Autodesk Inventor part; units mm, degrees
ref_plane "YZ Plane" through (0, 0, 0) normal (1, 0, 0) x (0, 1, 0)
ref_plane "XZ Plane" through (0, 0, 0) normal (0, 1, 0) x (-1, 0, 0)
ref_plane "XY Plane" through (0, 0, 0) normal (0, 0, 1) x (1, 0, 0)
sketch "草圖1" plane through (0, 0, 0) normal (0, 1, 0) x (-1, 0, 0)
  line L0 (-33.5, 27) -> (33.5, 27)
  line L1 (33.5, 27) -> (33.5, -27)
  line L2 (33.5, -27) -> (-33.5, -27)
  line L3 (-33.5, -27) -> (-33.5, 27)
  line L4 (-33.5, 27) -> (33.5, -27) construction
  line L5 (33.5, 27) -> (-33.5, -27) construction
  line L6 (43.5, -4.5) -> (33.5, -4.5)
  line L7 (33.5, -4.5) -> (33.5, 4.5)
  line L8 (33.5, 4.5) -> (43.5, 4.5)
  line L9 (43.5, 4.5) -> (43.5, -4.5)
  line L10 (-33.5, -4.5) -> (-43.5, -4.5)
  line L11 (-43.5, -4.5) -> (-43.5, 4.5)
  line L12 (-43.5, 4.5) -> (-33.5, 4.5)
  line L13 (-33.5, 4.5) -> (-33.5, -4.5)
  point P0 (0, 0)
  point P1 (33.5, 0)
  point P2 (-33.5, 0)
  point P3 (-33.5, 4.5)
  point P4 (-33.5, -4.5)
  dimension "d0" = 67
  dimension "d1" = 54
  dimension "d2" = 9
  dimension "d3" = 10
extrude "擠出1" add sketch "草圖1" along normal blind 450
sketch "草圖2" plane through (-33.5, 0, 27) normal (0, 0, 1) x (1, 0, 0)
  line L0 (0, 0) -> (0, 450)
  line L1 (0, 450) -> (67, 450)
  line L2 (67, 450) -> (67, 0)
  line L3 (67, 0) -> (0, 0)
  circle A0 centre (33.5, 225) radius 30
  line L4 (3.5, 225) -> (63.5, 225)
  line L5 (63.5, 225) -> (63.5, -27.0162)
  line L6 (63.5, -27.0162) -> (3.5, -27.0162)
  line L7 (3.5, -27.0162) -> (3.5, 225)
  point P0 (33.5, 0)
  point P1 (33.5, 0)
  point P2 (63.5, 225)
  point P3 (3.5, 225)
  dimension "d6" = 225
  dimension "d7" = 60
extrude "擠出2" cut sketch "草圖2" against normal through all contours L7 A0 L5 L3 | L3 L5 L6 L7 | L4 A0 | A0 L4
sketch "草圖3" plane through (-33.5, 450, 27) normal (0, 0, 1) x (1, 0, 0)
  line L0 (-76.6135, -320) -> (143.6135, -320)
  line L1 (143.6135, -320) -> (143.6135, -450)
  line L2 (143.6135, -450) -> (-76.6135, -450)
  line L3 (-76.6135, -450) -> (-76.6135, -320)
  point P0 (33.5, -450)
  point P1 (33.5, -450)
  dimension "d10" = 130
extrude "擠出3" cut sketch "草圖3" against normal through all
sketch "草圖4" plane through (33.5, 450, -27) normal (0, 0, -1) x (-1, 0, 0)
  arc A0 (63.5, -225) -> (3.5, -225) centre (33.5, -225) ccw construction
  circle A1 centre (33.5, -193) radius 30
  line L0 (63.5, -320) -> (3.5, -320)
  line L1 (3.5, -320) -> (3.5, -193)
  line L2 (3.5, -193) -> (63.5, -193)
  line L3 (63.5, -193) -> (63.5, -320)
  point P0 (33.5, -450)
  point P1 (63.5, -320)
  dimension "d13" = 32
  dimension "d14" = 60
sketch "草圖5" plane through (-33.5, 450, 27) normal (0, 0, 1) x (1, 0, 0)
  circle A0 centre (33.5, -191) radius 30
  arc A1 (63.5, -225) -> (3.5, -225) centre (33.5, -225) ccw construction
  line L0 (63.5, -320) -> (3.5, -320)
  line L1 (3.5, -320) -> (3.5, -191)
  line L2 (3.5, -191) -> (63.5, -191)
  line L3 (63.5, -191) -> (63.5, -320)
  point P0 (33.5, -450)
  point P1 (63.5, -320)
  dimension "d15" = 34
  dimension "d16" = 60
loft "斷面混成1" cut profiles "草圖4", "草圖5"
properties part number "Slider-9"
CAD build for the part. Positions are in the model's coordinates, mm. A direction names the side the tool comes from. Round coordinates to 2 decimals unless told otherwise and drop trailing zeros. Order: outer loops, then holes, each group sorted by start corner. A loop starts at its lowest first (then second) coordinate and runs counter-clockwise, first axis right, second up.
Q1. Drop flat-ended pins along their axis: pin 1 (10 mm diameter, centred on y = 392, z = -13, fed in from +X); pin 2 (11 mm diameter, centred on y = 350, z = 13.5, fed in from -X); pin 3 (3 mm diameter, centred on x = -37.5, y = 254.5, fed in from +Z). Give the stop position or say it passes through.
Q2. Slice it at C-C (x = -36.5). Write the cut outline in (y, z), and give its area (3 significant figures).
Q3. Which spindle directions (+Z, -Z, +X, -X, +Y, -Y) get a long thin tool onto all of the face, cutting with end or side? Do faces 4 (the flat face through (30, 195, 0)), 5 (the flat face through (-38, 288, 4.5)), 6 (the flat face through (-39, 288, -4.5)). Say none if no direction does.
Q4. Two-plate mould, pull along X, no slides. Class faces 1 (the flat face through (33.5, 288, -16)), 2 (the flat face through (0, 359, -27)), 3 (the flat face through (-30, 194, 0)): pulls with the +X half, pulls with the -X half, needs draft (parallel to the pull), parting line crosses it, or undercut.
Q5. Slice it at A-A (y = 215). Write the cut outline in (x, z).
Q6. Wall check: L1, parallel to X at y = 217.5, z = 11.5; L2, parallel to X at y = 332, z = 10; L3, parallel to Z at x = -39.5, y = 374.5. Give the ranges that are in metal, low to high.
Q7. Slice it at B-B (y = 292.5). Write the cut outline in (x, z), and give its area (3 significant figures).
Results below:
1. pin 1: stops at x = 33.5
1. pin 2: stops at x = -33.5
1. pin 3: stops at z = 4.5
2. outline: (130, -4.5) - (450, -4.5) - (450, 4.5) - (130, 4.5) - close
2. area: 2,880 mm2
3. face 4: +Z, -Z, -Y
3. face 5: +Z, -X, +Y, -Y
3. face 6: -Z, -X, +Y, -Y
4. face 1: pulls with the +X half
4. face 2: needs draft
4. face 3: undercut
5. outline: (-43.5, -4.5) - (-33.5, -4.5) - (-33.5, -27) - (-30, -27) - (-30, 27) - (-33.5, 27) - (-33.5, 4.5) - (-43.5, 4.5) - close; (30, -27) - (33.5, -27) - (33.5, -4.5) - (43.5, -4.5) - (43.5, 4.5) - (33.5, 4.5) - (33.5, 27) - (30, 27) - close
6. L1: x = -33.5 to -30, 30 to 33.5
6. L2: x = -33.5 to 33.5
6. L3: z = -4.5 to 4.5
7. outline: (-43.5, -4.5) - (-33.5, -4.5) - (-33.5, -27) - (33.5, -27) - (33.5, -4.5) - (43.5, -4.5) - (43.5, 4.5) - (33.5, 4.5) - (33.5, 27) - (-33.5, 27) - (-33.5, 4.5) - (-43.5, 4.5) - close
7. area: 3,800 mm2
